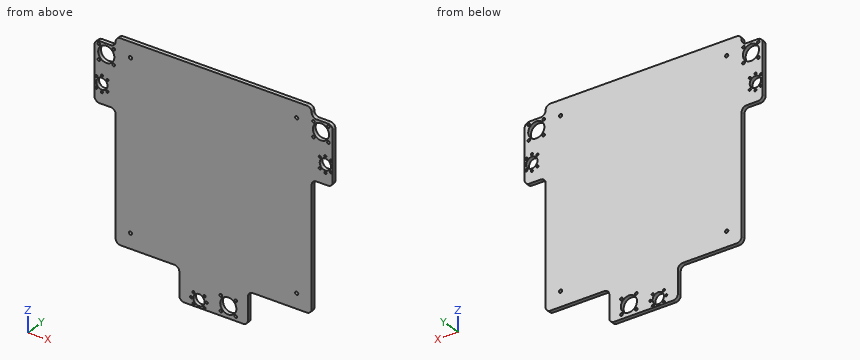
from build123d import *

# Parameters (mm, degrees)
SKETCH2_W            = 486
SKETCH2_H            = 446
BOSS_EXTRUDE1_DEPTH  = 8
M5_CLEARANCE_HOLE1_D = 5.5
M4_CLEARANCE_HOLE1_D = 4.5
SKETCH8_R            = 11.5
SKETCH8_R_2          = 16.5
CUT_EXTRUDE1_DEPTH   = 346.874254607
M5_CLEARANCE_HOLE2_D = 5.5
M4_CLEARANCE_HOLE2_D = 4.5
SKETCH13_R           = 11.5
SKETCH13_R_2         = 16.5
CUT_EXTRUDE2_DEPTH   = 346.874254607
CUT_EXTRUDE5_DEPTH   = 346.874254607
SKETCH20_W           = 400
SKETCH20_H           = 400
BOSS_EXTRUDE2_DEPTH  = 8
FILLET3_R            = 10
M6_CLEARANCE_HOLE1_D = 6.6


with BuildPart() as part:
    # Sketch2 → Boss-Extrude1 (new body)
    with BuildSketch(Plane(origin=(0, 0, 0), x_dir=(1, 0, 0), z_dir=(0, 1, 0))):
        with Locations((0, 23)):
            Rectangle(SKETCH2_W, SKETCH2_H)
    extrude(amount=BOSS_EXTRUDE1_DEPTH)

    # M5 Clearance Hole1 (through all)
    with Locations(Plane(origin=(0, 8, 0), x_dir=(1, 0, 0), z_dir=(0, 1, 0))):
        with Locations((-234.202795796, -163.797204204), (-203.797204204, -163.797204204), (-203.797204204, -194.202795796), (-234.202795796, -194.202795796)):
            m5_clearance_hole1 = Hole(M5_CLEARANCE_HOLE1_D / 2)

    # M4 Clearance Hole1 (through all)
    with Locations(Plane(origin=(0, 8, 0), x_dir=(1, 0, 0), z_dir=(0, 1, 0))):
        with Locations((-228, -135), (-216.686291501, -130.313708499), (-216.686291501, -107.686291501), (-228, -103), (-239.313708499, -107.686291501), (-239.313708499, -130.313708499)):
            m4_clearance_hole1 = Hole(M4_CLEARANCE_HOLE1_D / 2)

    # Sketch8 → Cut-Extrude1 (cut, through all)
    with BuildSketch(Plane(origin=(0, 8, 0), x_dir=(1, 0, 0), z_dir=(0, 1, 0))):
        with Locations(Location((-228, -119, 0), (0, 0, 270))):
            Circle(SKETCH8_R)
        with Locations(Location((-219, -179, 0), (0, 0, 270))):
            Circle(SKETCH8_R_2)
    cut_extrude1 = extrude(amount=-CUT_EXTRUDE1_DEPTH, mode=Mode.SUBTRACT)

    # Mirror1: M5 Clearance Hole1, M4 Clearance Hole1, Cut-Extrude1 across plane
    add(m5_clearance_hole1.mirror(Plane(origin=(0, 0, 0), x_dir=(0, 0, 1), z_dir=(1, 0, 0))), mode=Mode.SUBTRACT)
    add(m4_clearance_hole1.mirror(Plane(origin=(0, 0, 0), x_dir=(0, 0, 1), z_dir=(1, 0, 0))), mode=Mode.SUBTRACT)
    add(cut_extrude1.mirror(Plane(origin=(0, 0, 0), x_dir=(0, 0, 1), z_dir=(1, 0, 0))), mode=Mode.SUBTRACT)

    # M5 Clearance Hole2 (through all)
    with Locations(Plane(origin=(0, 8, 0), x_dir=(1, 0, 0), z_dir=(0, 1, 0))):
        with Locations((45.202795796, 206.797204204), (14.797204204, 206.797204204), (14.797204204, 237.202795796), (45.202795796, 237.202795796)):
            Hole(M5_CLEARANCE_HOLE2_D / 2)

    # M4 Clearance Hole2 (through all)
    with Locations(Plane(origin=(0, 8, 0), x_dir=(1, 0, 0), z_dir=(0, 1, 0))):
        with Locations((-41.313708499, 219.686291501), (-46, 231), (-41.313708499, 242.313708499), (-18.686291501, 242.313708499), (-14, 231), (-18.686291501, 219.686291501)):
            Hole(M4_CLEARANCE_HOLE2_D / 2)

    # Sketch13 → Cut-Extrude2 (cut, through all)
    with BuildSketch(Plane(origin=(0, 8, 0), x_dir=(1, 0, 0), z_dir=(0, 1, 0))):
        with Locations(Location((-30, 231, 0), (0, 0, 270))):
            Circle(SKETCH13_R)
        with Locations(Location((30, 222, 0), (0, 0, 270))):
            Circle(SKETCH13_R_2)
    extrude(amount=-CUT_EXTRUDE2_DEPTH, mode=Mode.SUBTRACT)

    # Sketch19 → Cut-Extrude5 (cut, through all)
    with BuildSketch(Plane(origin=(0, 8, 0), x_dir=(1, 0, 0), z_dir=(0, 1, 0))):
        Polygon((-243, -80), (-200, -80), (-200, 180), (-70, 180), (-70, 246), (-243, 246), align=None)
    cut_extrude5 = extrude(amount=-CUT_EXTRUDE5_DEPTH, mode=Mode.SUBTRACT)

    # Mirror2: Cut-Extrude5 across plane
    add(cut_extrude5.mirror(Plane(origin=(0, 0, 0), x_dir=(0, 0, 1), z_dir=(1, 0, 0))), mode=Mode.SUBTRACT)

    # Sketch20 → Boss-Extrude2 (add)
    with BuildSketch(Plane(origin=(0, 8, 0), x_dir=(1, 0, 0), z_dir=(0, 1, 0))):
        with Locations((0, -20)):
            Rectangle(SKETCH20_W, SKETCH20_H)
    extrude(amount=-BOSS_EXTRUDE2_DEPTH)

    # Fillet3
    fillet3_edges = [part.edges().sort_by_distance(p)[0] for p in [
        (-243, 4, 80),
        (-70, 4, -246),
        (-70, 4, -180),
        (-200, 4, -180),
        (-200, 4, 80),
        (243, 4, 80),
        (200, 4, 80),
        (200, 4, -180),
        (70, 4, -180),
        (70, 4, -246),
        (-200, 4, 220),
        (200, 4, 200),
        (-200, 4, 200),
        (200, 4, 220),
        (243, 4, 200),
        (-243, 4, 200),
    ]]
    fillet(fillet3_edges, radius=FILLET3_R - 0.0001)  # a hair under: the kernel refuses the full size

    # M6 Clearance Hole1 (through all)
    with Locations(Plane(origin=(0, 8, 0), x_dir=(1, 0, 0), z_dir=(0, 1, 0))):
        with Locations((-169.5, -189.5), (-169.5, 149.5), (169.5, 149.5), (169.5, -189.5)):
            Hole(M6_CLEARANCE_HOLE1_D / 2)


solid = part.part
Check sheet for the modelled part. Datum: model origin and axes. Units: mm. Round coordinates to 2 decimals unless told otherwise and drop trailing zeros. Order: outer loops, then holes, each group sorted by start corner. A loop starts at its lowest first (then second) coordinate and runs counter-clockwise, first axis right, second up.
(1) Cross-section at B-B, the plane z = 116.5. Enter the section's corners in (x, y).
(2) Cross-section at D-D, the plane y = 2.25. State how many separate pieces and enclosed holes the cut face has, and give its area (3 significant figures).
(3) Scan lines: probe 1 along X at (y, z) = (6.25, 119); probe 2 along Z at (x, y) = (-14, 4); probe 3 along Z at (x, y) = (-169.5, 4.5). Record each from-to range of solid material in increasing order.
(4) Cross-section at A-A, the plane x = 30. Enter the section's corners in (y, z).
(5) Cross-section at C-C, the plane z = 50.5. Enter the section's corners in (x, y), and give its area (3 significant figures).
(6) Go/stop test with flat-tipped pins: P1, Ø2.5, axis at x = 111, y = 6, coming from the -Z side; P2, Ø2.5, axis at y = 5.5, z = -216, coming from the +X side; P3, Ø4, axis at y = 6.5, z = -188.5, coming from the +X side; P4, Ø6, axis at x = -169.5, z = -149.5, coming from the +Y side. Record where each tip stops, or that it passes through.
Check sheet entries:
1. outline: (-243, 0) - (-239.22, 0) - (-239.22, 8) - (-243, 8) - close; (-216.78, 0) - (216.78, 0) - (216.78, 8) - (-216.78, 8) - close; (239.22, 0) - (243, 0) - (243, 8) - (239.22, 8) - close
2. separate pieces: 1
2. enclosed holes: 40
2. area: 175,000 mm2
3. probe 1: x = -243 to -239.5, -216.5 to 216.5, 239.5 to 243
3. probe 2: z = -246 to -233.25, -228.75 to 220
3. probe 3: z = -180 to -152.8, -146.2 to 186.2, 192.8 to 220
4. outline: (0, -246) - (8, -246) - (8, -238.5) - (0, -238.5) - close; (0, -205.5) - (8, -205.5) - (8, 220) - (0, 220) - close
5. outline: (-200, 0) - (200, 0) - (200, 8) - (-200, 8) - close
5. area: 3,200 mm2
6. P1: stops at z = -180
6. P2: stops at x = 70
6. P3: stops at x = 70.63
6. P4: passes through
